from build123d import *

# Parameters (mm, degrees)
BOSS_EXTRUDE1_DEPTH   = 2.5
SKETCH2_W             = 7
SKETCH2_H             = 2.5
BOSS_EXTRUDE2_DEPTH   = 9.5
CUT_EXTRUDE1_DEPTH    = 9.5
SKETCH4_R             = 1.275
CUT_EXTRUDE2_DEPTH    = 9.5
M2X0_4_TAPPED_HOLE1_D = 1.6
FILLET1_R             = 0.2


with BuildPart() as part:
    # Sketch1 → Boss-Extrude1 (new body, symmetric)
    with BuildSketch(Plane(origin=(0, 0, 0), x_dir=(1, 0, 0), z_dir=(0, 1, 0))):
        with BuildLine():
            Line((1.96, 0), (8, 0))
            ThreePointArc((8, 0), (0, -8), (-8, 0))
            Line((-8, 0), (-1.96, 0))
            ThreePointArc((-1.96, 0), (0, -1.96), (1.96, 0))
        make_face()
    extrude(amount=BOSS_EXTRUDE1_DEPTH, both=True)

    # Sketch2 → Boss-Extrude2 (add)
    with BuildSketch(Plane(origin=(0, 2.5, 0), x_dir=(1, 0, 0), z_dir=(0, 1, 0))):
        with Locations((0, -5)):
            Rectangle(SKETCH2_W, SKETCH2_H)
    extrude(amount=BOSS_EXTRUDE2_DEPTH)

    # Sketch3 → Cut-Extrude1 (cut)
    with BuildSketch(Plane(origin=(0, 0, 3.75), x_dir=(-1, 0, 0), z_dir=(0, 0, -1))):
        with BuildLine():
            Line((-3.5, 8.5), (-3.5, 14.886359519))
            Line((-3.5, 14.886359519), (0, 16.809201746))
            Line((0, 16.809201746), (3.5, 14.5))
            Line((3.5, 14.5), (3.5, 8.5))
            ThreePointArc((3.5, 8.5), (0, 12), (-3.5, 8.5))
        make_face()
    extrude(amount=-CUT_EXTRUDE1_DEPTH, mode=Mode.SUBTRACT)

    # Sketch4 → Cut-Extrude2 (cut)
    with BuildSketch(Plane(origin=(0, 0, 3.75), x_dir=(-1, 0, 0), z_dir=(0, 0, -1))):
        with Locations((0, 8.5)):
            Circle(SKETCH4_R)
    extrude(amount=-CUT_EXTRUDE2_DEPTH, mode=Mode.SUBTRACT)

    # M2x0.4 Tapped Hole1 (through all)
    with Locations(Plane(origin=(0, 0, 0), x_dir=(-1, 0, 0), z_dir=(0, 0, -1))):
        with Locations((-5, 0), (5, 0)):
            Hole(M2X0_4_TAPPED_HOLE1_D / 2)

    # Fillet1
    fillet1_edges = [part.edges().sort_by_distance(p)[0] for p in [
        (1.96, 0, 0),
        (-1.96, 0, 0),
    ]]
    fillet(fillet1_edges, radius=FILLET1_R)


solid = part.part
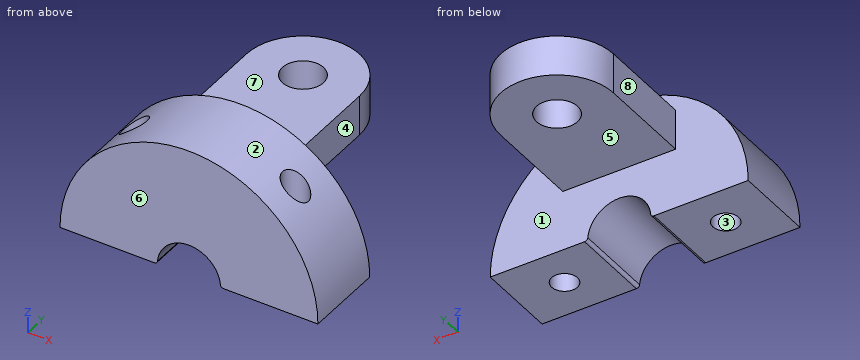
Design review of the part built by this model. Coordinates are the model's own, in mm. Face numbers are marked on the shaded views. A direction names the side the tool comes from. Round coordinates to 2 decimals unless told otherwise and drop trailing zeros. Write each loop counter-clockwise with the first axis right and the second up, starting at its lowest first coordinate (ties: lowest second). Pieces come first, ordered by that corner, then holes. Notation, with made-up numbers: (62.5, 61) -> (113.5, 61) arc R5 ccw to (113.5, 65) -> close; hole circle Ø6 at (-2, 5). An arc over 180 degrees is marked (long way). One line per item, written item: value. Start each with the question number.
Q1. Insertion check: P1, Ø2, axis at x = -5.5, z = 7, coming from the +Y side; P2, Ø1.5, axis at x = -6, y = 0, coming from the +Z side; P3, Ø1.2, axis at y = 6.5, z = 5.5, coming from the +X side. Each pin has a flat end and moves straight along its axis. Give the tip position at first contact, or say it passes through.
Q2. Tool access review of the marked faces 4, 5, 6, 7 and 8: name each direction out of +Z, -Z, +X, -X, +Y, -Y from which nothing blocks a thin tool from reaching the whole face with its end or side.
Q3. Add section B-B (y = -0.5). Give the boundary of the cut face in (x, z).
Q4. To check wall thickness, follow probe 1 along Y at (x, z) = (-5, 3.5); probe 2 along X at (y, z) = (0, 3.25); probe 3 along Y at (x, z) = (0, 5.55) (3 decimals). State the ranges of each line that lie inside material, in increasing order.
Q5. The part is to be moulded in two halves that separate along X. For the marked faces 1, 2 and 3, say which applies: pulls with the +X half, pulls with the -X half, needs draft (parallel to the pull), parting line crosses it, or undercut.
Q6. Add section A-A (z = 1.5). Give the boundary of the cut face in (x, y), then the cut area to 3 significant figures.
Q7. Add section C-C (x = 0). Give the boundary of the cut face in (y, z) (3 decimals).
Response:
1. P1: stops at y = 2.5
1. P2: stops at z = 5.77
1. P3: stops at x = 3.5
2. face 4: +Z, -Z, +X, +Y
2. face 5: -Z, +X, -X, +Y
2. face 6: +Z, -Z, +X, -X, -Y
2. face 7: +Z, +X, -X, +Y
2. face 8: +Z, -Z, -X, +Y
3. outline: (-8, 0) -> (-5.62, 0) -> (-5.62, 5.69) arc R8 ccw to start; (-4.38, 0) -> (-2.15, 0) arc R0.2 ccw to (-1.95, 0.18) arc R1.96 cw to (1.95, 0.18) arc R0.2 ccw to (2.15, 0) -> (4.38, 0) -> (4.38, 6.7) arc R8 ccw to (-4.38, 6.7) -> close; (5.62, 0) -> (8, 0) arc R8 ccw to (5.62, 5.69) -> close
4. probe 1: y = -2.5 to -0.8, 0.8 to 2.5
4. probe 2: x = -7.31 to -5.8, -4.2 to 4.2, 5.8 to 7.31
4. probe 3: y = -2.5 to 7.225, 9.775 to 12
5. face 1: needs draft
5. face 2: parting line crosses it
5. face 3: undercut
6. outline: (-7.86, -2.5) -> (-1.26, -2.5) -> (-1.26, 2.5) -> (-7.86, 2.5) -> close; (1.26, -2.5) -> (7.86, -2.5) -> (7.86, 2.5) -> (1.26, 2.5) -> close; hole circle Ø1.6 at (-5, 0); hole circle Ø1.6 at (5, 0)
6. area: 61.9 mm^2
7. outline: (-2.5, 1.96) -> (2.5, 1.96) -> (2.5, 3.75) -> (7.225, 3.75) -> (7.225, 6.25) -> (2.5, 6.25) -> (2.5, 8) -> (-2.5, 8) -> close; (9.775, 3.75) -> (12, 3.75) -> (12, 6.25) -> (9.775, 6.25) -> close
